Check sheet for the modelled part. Datum: model origin and axes. Units: mm. A direction names the side the tool comes from. Give positions to 0.01 mm unless a question says otherwise; leave off trailing zeros. Order: outer loops, then holes, each group sorted by start corner. A loop starts at its lowest first (then second) coordinate and runs counter-clockwise, first axis right, second up. Notation, with made-up numbers: (-22.5, 50) -> (23.5, 50) arc R20 ccw to (23.5, 74) -> close; hole circle Ø10 at (7.5, 48). An arc over 180 degrees is marked (long way). Answer in a Markdown table with one row per item. Add a question column.
(1) Set-up check for faces 1 (the face through (0.834, -1, -1)), 2 (the face through (2, -4.16, 0.63)), 3 (the face through (-0.33, -0.97, 2.52)): record each of +Z, -Z, +X, -X, +Y, -Y from which the full face is reachable in a straight line by a thin tool's end or side.
(2) Thickness scan on L1, parallel to Z at x = 0.1, y = -0.25; L2, parallel to Y at x = -0.9, z = 0; L3, parallel to Y at x = 2.2, z = -0.95 (3 decimals). Record the ranges inside material, lowest first. Write a range as [from, to].
(3) Go/stop test with flat-tipped pins: pin 1 (2 mm diameter, centred on x = -1, y = -2.5, fed in from +Z); pin 2 (1 mm diameter, centred on y = -0.5, z = -1.5, fed in from +X); pin 3 (1 mm diameter, centred on x = 1.5, y = -0.5, fed in from -Z). Record where each tip stops, or that it passes through.
(4) Cross-section at C-C (y = -3.25). Record the cut outline in (x, z).
Autodesk Inventor part; units mm, degrees
ref_plane "YZ Plane" through (0, 0, 0) normal (1, 0, 0) x (0, 1, 0)
ref_plane "XZ Plane" through (0, 0, 0) normal (0, 1, 0) x (-1, 0, 0)
ref_plane "XY Plane" through (0, 0, 0) normal (0, 0, 1) x (1, 0, 0)
sketch "Sketch1" plane through (0, 0, 0) normal (0, 0, 1) x (1, 0, 0)
  line L0 (0, 0) -> (2.54, 0)
  line L1 (2.54, 0) -> (2.54, -1.905)
  line L2 (2.54, -1.905) -> (2.0955, -1.905)
  line L3 (2.0955, -1.905) -> (2.0955, -6.35)
  line L4 (2.0955, -6.35) -> (0, -6.35)
  line L5 (0, -6.35) -> (0, 0)
  line L6 (0, 0) -> (0, -8.8327)
  dimension "d0" = 2.54
  dimension "d1" = 1.905
  dimension "d2" = 0.4445
  dimension "d3" = 4.445
revolve "Revolution1" add sketch "Sketch1" angle 360 about axis through (0, 0, 0) along (0, -1, 0)
thread "Thread1"
sketch "Sketch2" plane through (0, 0, 0) normal (0, 1, 0) x (1, 0, 0)
  line L0 (2.1608, 0.7916) -> (2.1608, -1.0055)
  line L1 (-2.1181, -1.0055) -> (-2.1181, 0.7916)
  line L2 (-0.7916, 2.0955) -> (0.8344, 2.0955)
  line L3 (0.8344, -2.2464) -> (-0.7916, -2.2464)
  line L4 (-0.7916, -2.2464) -> (-0.7916, -1.0055)
  line L5 (-0.7916, 0.7916) -> (-0.7916, 2.0955)
  line L6 (-2.1181, 0.7916) -> (-0.7916, 0.7916)
  line L7 (0.8344, 0.7916) -> (2.1608, 0.7916)
  line L8 (0.8344, 2.0955) -> (0.8344, 0.7916)
  line L9 (0.8344, -1.0055) -> (0.8344, -2.2464)
  line L10 (2.1608, -1.0055) -> (0.8344, -1.0055)
  line L11 (-0.7916, -1.0055) -> (-2.1181, -1.0055)
  point P0 (0, 0)
extrude "Extrusion1" cut sketch "Sketch2" against normal blind 1.27
properties part number "sqrew for baring stand" material "Aluminum 6061"
Answer below:
| question | item | result |
|---|---|---|
| 1 | face 1 | +Y |
| 1 | face 2 | -Y |
| 1 | face 3 | +Y, -Y |
| 2 | L1 | z = [-2.54, -2.1], [2.25, 2.54] |
| 2 | L2 | y = [-6.35, -1.27] |
| 2 | L3 | y = [-1.905, 0] |
| 3 | pin 1 | stops at z = 2.53 |
| 3 | pin 2 | stops at x = 2.33 |
| 3 | pin 3 | stops at z = -2.33 |
| 4 | outline | circle Ø4.19 at (0, 0) |
